```python
from build123d import *

# Parameters (mm, degrees)
CROQUIS1_W                    = 27
CROQUIS1_H                    = 23.199
SALIENTE_EXTRUIR1_DEPTH       = 10
CORTAR_EXTRUIR1_DEPTH         = 30.823541054
CROQUIS3_W                    = 0.55
CROQUIS3_H                    = 4.9
CORTAR_EXTRUIR2_DEPTH         = 30.823541054
CORTAR_EXTRUIR3_DEPTH         = 30.823541054
CORTAR_EXTRUIR4_DEPTH         = 23.199
CROQUIS6_W                    = 0.55
CROQUIS6_H                    = 4.9
CORTAR_EXTRUIR5_DEPTH         = 30.823541054
CROQUIS7_W                    = 10
CROQUIS7_H                    = 0.2
CORTAR_EXTRUIR6_DEPTH         = 30.823541054
DI_METRO_DE_TALADRO_1_0_1_1_D = 1
CHAFL_N1_SIZE                 = 0.305
CHAFL_N2_SIZE                 = 0.6


with BuildPart() as part:
    # Croquis1 → Saliente-Extruir1 (new body)
    with BuildSketch(Plane.XY.offset(13)):
        with Locations((0, 74.9)):
            Rectangle(CROQUIS1_W, CROQUIS1_H)
    extrude(amount=-SALIENTE_EXTRUIR1_DEPTH)

    # Croquis2 → Cortar-Extruir1 (cut, through all)
    with BuildSketch(Plane.XZ.offset(-63.3005)):
        with BuildLine():
            Line((-5.125, 3), (5.125, 3))
            Line((5.125, 3), (5.125, 6.799999997))
            ThreePointArc((5.125, 6.799999997), (5.375, 7.461437825), (6, 7.79215674))
            Line((6, 7.79215674), (6, 8.6))
            Line((6, 8.6), (-6, 8.6))
            Line((-6, 8.6), (-6, 7.79215674))
            ThreePointArc((-6, 7.79215674), (-5.375, 7.461437828), (-5.125, 6.800000001))
            Line((-5.125, 6.800000001), (-5.125, 3))
        make_face()
    extrude(amount=-CORTAR_EXTRUIR1_DEPTH, mode=Mode.SUBTRACT)

    # Croquis3 → Cortar-Extruir2 (cut, through all)
    with BuildSketch(Plane.XZ.offset(-63.3005)):
        with Locations((13.225, 5.45)):
            Rectangle(CROQUIS3_W, CROQUIS3_H)
    extrude(amount=-CORTAR_EXTRUIR2_DEPTH, mode=Mode.SUBTRACT)

    # Croquis4 → Cortar-Extruir3 (cut, through all)
    with BuildSketch(Plane.XZ.offset(-63.3005)):
        with BuildLine():
            Line((5.125, 4.199999999), (5.125, 3))
            Line((5.125, 3), (6, 3))
            Line((6, 3), (6, 3.20784326))
            ThreePointArc((6, 3.20784326), (5.375, 3.538562172), (5.125, 4.199999999))
        make_face()
    extrude(amount=-CORTAR_EXTRUIR3_DEPTH, mode=Mode.SUBTRACT)

    # Croquis5 → Cortar-Extruir4 (cut)
    with BuildSketch(Plane.XZ.offset(-63.3005)):
        with BuildLine():
            Line((-6, 3.20784326), (-6, 3))
            Line((-6, 3), (-5.125, 3))
            Line((-5.125, 3), (-5.125, 4.200000003))
            ThreePointArc((-5.125, 4.200000003), (-5.375, 3.538562175), (-6, 3.20784326))
        make_face()
    extrude(amount=-CORTAR_EXTRUIR4_DEPTH, mode=Mode.SUBTRACT)

    # Croquis6 → Cortar-Extruir5 (cut, through all)
    with BuildSketch(Plane.XZ.offset(-63.3005)):
        with Locations((-13.225, 5.45)):
            Rectangle(CROQUIS6_W, CROQUIS6_H)
    extrude(amount=-CORTAR_EXTRUIR5_DEPTH, mode=Mode.SUBTRACT)

    # Croquis7 → Cortar-Extruir6 (cut, through all)
    with BuildSketch(Plane.XZ.offset(-63.3005)):
        with Locations((0, 12.9)):
            Rectangle(CROQUIS7_W, CROQUIS7_H)
    extrude(amount=-CORTAR_EXTRUIR6_DEPTH, mode=Mode.SUBTRACT)

    # Croquis8 → Cortar-Revolución1 (revolve, cut)
    with BuildSketch(Plane.XZ.offset(-67.4), mode=Mode.PRIVATE) as cortar_revoluci_n1_sk:
        Polygon((-8.805, 13), (-10, 13), (-10, 8.307179677), (-8.8, 9), (-8.8, 9.5), (-8.805, 9.5), align=None)
    revolve(cortar_revoluci_n1_sk.sketch.rotate(Axis((-10, 67.4, 13.000025), (0, 0, -1)), 180), axis=Axis((-10, 67.4, 13.000025), (0, 0, -1)), mode=Mode.SUBTRACT)

    # Croquis9 → Cortar-Revolución2 (revolve, cut)
    with BuildSketch(Plane.XZ.offset(-82.4), mode=Mode.PRIVATE) as cortar_revoluci_n2_sk:
        Polygon((-8.805, 13), (-10, 13), (-10, 8.307179677), (-8.8, 9), (-8.8, 9.5), (-8.805, 9.5), align=None)
    revolve(cortar_revoluci_n2_sk.sketch.rotate(Axis((-10, 82.4, 13.000025), (0, 0, -1)), 180), axis=Axis((-10, 82.4, 13.000025), (0, 0, -1)), mode=Mode.SUBTRACT)

    # Croquis10 → Cortar-Revolución3 (revolve, cut)
    with BuildSketch(Plane.XZ.offset(-67.4), mode=Mode.PRIVATE) as cortar_revoluci_n3_sk:
        Polygon((11.195, 13), (10, 13), (10, 8.307179677), (11.2, 9), (11.2, 9.5), (11.195, 9.5), align=None)
    revolve(cortar_revoluci_n3_sk.sketch.rotate(Axis((10, 67.4, 13.000025), (0, 0, -1)), 180), axis=Axis((10, 67.4, 13.000025), (0, 0, -1)), mode=Mode.SUBTRACT)

    # Croquis11 → Cortar-Revolución4 (revolve, cut)
    with BuildSketch(Plane.XZ.offset(-82.4), mode=Mode.PRIVATE) as cortar_revoluci_n4_sk:
        Polygon((11.195, 13), (10, 13), (10, 8.307179677), (11.2, 9), (11.2, 9.5), (11.195, 9.5), align=None)
    revolve(cortar_revoluci_n4_sk.sketch.rotate(Axis((10, 82.4, 13.000025), (0, 0, -1)), 180), axis=Axis((10, 82.4, 13.000025), (0, 0, -1)), mode=Mode.SUBTRACT)

    # Diámetro de taladro Ø1.0 (1)1 (through all)
    with Locations(Plane(origin=(0, 86.4995, 0), x_dir=(-1, 0, 0), z_dir=(0, 1, 0))):
        with Locations((-13.5, 10.3)):
            Hole(DI_METRO_DE_TALADRO_1_0_1_1_D / 2)

    # Chaflán1
    chafl_n1_edges = [part.edges().sort_by_distance(p)[0] for p in [
        (-8.805, 67.4, 13),
        (-8.805, 82.4, 13),
        (11.195, 67.4, 13),
        (11.195, 82.4, 13),
    ]]
    chamfer(chafl_n1_edges, length=CHAFL_N1_SIZE)

    # Chaflán2
    chafl_n2_edges = [part.edges().sort_by_distance(p)[0] for p in [
        (13.5, 74.9, 13),
        (-13.5, 74.9, 13),
    ]]
    chamfer(chafl_n2_edges, length=CHAFL_N2_SIZE)


solid = part.part
```
Source: CAD feature listing. Evaluate the final solid. Frame: model axes, mm. A direction names the side the tool comes from. Coordinates: 2 decimals unless noted, no trailing zeros. Order: outer loops, then holes, each group sorted by start corner. A loop starts at its lowest first (then second) coordinate and runs counter-clockwise, first axis right, second up. Notation, with made-up numbers: M 58.5,-39 L 67.5,-39 A15 cw 67.5,-26 Z; hole C -14,-28.5 d6. An arc over 180 degrees is marked long. Write each question's results on one line, items separated by ' | '. Start each with the question number.
1) Line query: line 1 (X direction, y = 82.4, z = 9.45); line 2 (Y direction, x = -10, z = 11.7) (1 decimal); line 3 (Z direction, x = -3.5, y = 69.5). Output: solid intervals per line, ascending. Write a range as from..to.
2) Section query B-B (y = 65.5). Return the cut outline in (x, z) (3 decimals).
3) Section query A-A (z = 11.5). Return the cut outline in (x, y) (1 decimal).
4) Access query for faces 1 (the face through (12.95, 75, 5)), 2 (the face through (0, 75, 12.8)), 3 (the face through (-5.38, 74.74, 7.47)), 4 (the face through (-5.125, 75, 6)). Directions: +Z, -Z, +X, -X, +Y, -Y. A direction counts if a zero-diameter tool reaches every point of the face in a straight line with its end or side. Return the directions, or none.
5) Contact query for flat-ended pins moving along their axis: pin 1 Ø1.9 at (x, y) = (10, 82.4) entering from +Z; pin 2 Ø4 at (x, y) = (-10, 82.4) entering from +Z; pin 3 Ø6 at (x, y) = (-1, 76) entering from -Z; pin 4 Ø2 at (y, z) = (71.5, 5) entering from -X. Output: stop coordinate, or through.
6) Draft query along Y for faces 5 (the face through (9, 75, 3)), 6 (the face through (9.904, 82.215, 8.427)). Return one class per face: released by +Y, released by -Y, zero draft, split by the parting line, or undercut.
7) Section query C-C (x = 3.5). Return the cut outline in (y, z), plus the area to 3 significant figures.
Answers:
1) line 1: x = -13.5..-11.2, -8.8..8.8, 11.2..13.5 | line 2: y = 63.3..66.2, 68.6..81.2, 83.6..86.5 | line 3: z = 8.6..12.8
2) outline: M -13.5,7.9 L -12.95,7.9 L -12.95,3 L -6,3 L -6,3.208 A1 ccw -5.125,4.2 L -5.125,6.8 A1 ccw -6,7.792 L -6,8.6 L 6,8.6 L 6,7.792 A1 ccw 5.125,6.8 L 5.125,4.2 A1 ccw 6,3.208 L 6,3 L 12.95,3 L 12.95,7.9 L 13.5,7.9 L 13.5,9.8 A0.5 cw 13.5,10.8 L 13.5,12.4 L 12.9,13 L 5,13 L 5,12.8 L -5,12.8 L -5,13 L -12.9,13 L -13.5,12.4 Z
3) outline: M -13.5,63.3 L 13.5,63.3 L 13.5,86.5 L -13.5,86.5 Z; hole C -10,67.4 d2.4; hole C -10,82.4 d2.4; hole C 10,67.4 d2.4; hole C 10,82.4 d2.4
4) face 1: -Z, +X, +Y, -Y | face 2: +Z, +Y, -Y | face 3: +Y, -Y | face 4: -Z, +Y, -Y
5) pin 1: stops at z = 8.86 | pin 2: stops at z = 13 | pin 3: stops at z = 8.6 | pin 4: stops at x = -12.95
6) face 5: zero draft | face 6: undercut
7) outline: M 63.3,8.6 L 86.5,8.6 L 86.5,12.8 L 63.3,12.8 Z | area: 97.4 mm^2
